Geometry check sheet. Reference: the model listing, model coordinates, mm. Face numbers are marked on the shaded views. Round coordinates to 2 decimals unless told otherwise and drop trailing zeros. Loops run counter-clockwise (first coordinate to the right, second up) from the corner with the lowest first, then second, coordinate; pieces in that order, holes last. Notation, with made-up numbers: (-23, -4.5) -> (-17, -4.5) arc R24 ccw to (-17, 24.5) -> close; hole circle Ø3 at (-8, 45.25). An arc over 180 degrees is marked (long way). Use a Markdown table: item, result. Add a question column.
Q1. Sectioned sample at B-B, the plane z = 4.25. Enter the section's corners in (x, y), then the cut area to 3 significant figures.
Q2. Sectioned sample at C-C, the plane x = 0. Enter the section's corners in (y, z).
Q3. Release check for a two-part mould opening along X. For the marked faces 1, 2 and 3 record: released by +X, released by -X, zero draft, split by the parting line, or undercut.
Q4. Sectioned sample at D-D, the plane x = 2. Enter the section's corners in (y, z), then the cut area to 3 significant figures.
Q5. Material ranges on L1, parallel to Y at x = 0, z = 1.15; L2, parallel to X at y = -12, z = 2.8; L3, parallel to X at y = 9, z = 0.45, recorded low to high.
Q6. Sectioned sample at A-A, the plane y = -10. Enter the section's corners in (x, z).
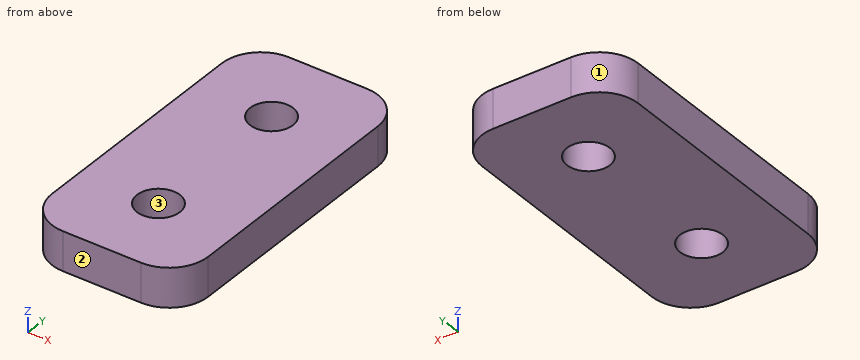
```python
from build123d import *

# Parameters (mm, degrees)
F0_W     = 20
F0_H     = 40
F0_R     = 2.75
F1_DEPTH = 5
F2_R     = 5


with BuildPart() as f1:
    # F0 (on Top) → F1 (new body)
    with BuildSketch(Plane.XY):
        Rectangle(F0_W, F0_H)
        with Locations((0, -10)):
            Circle(F0_R, mode=Mode.SUBTRACT)
        with Locations((0, 10)):
            Circle(F0_R, mode=Mode.SUBTRACT)
    extrude(amount=F1_DEPTH)

    # F2
    f2_edges = [f1.edges().sort_by_distance(p)[0] for p in [
        (-10, 20, 2.5),
        (10, 20, 2.5),
        (10, -20, 2.5),
        (-10, -20, 2.5),
    ]]
    fillet(f2_edges, radius=F2_R)


solid = f1.part
```
Values:
| question | item | result |
|---|---|---|
| 1 | outline | (-10, -15) arc R5 ccw to (-5, -20) -> (5, -20) arc R5 ccw to (10, -15) -> (10, 15) arc R5 ccw to (5, 20) -> (-5, 20) arc R5 ccw to (-10, 15) -> close; hole circle Ø5.5 at (0, -10); hole circle Ø5.5 at (0, 10) |
| 1 | area | 731 mm^2 |
| 2 | outline | (-20, 0) -> (-12.75, 0) -> (-12.75, 5) -> (-20, 5) -> close; (-7.25, 0) -> (7.25, 0) -> (7.25, 5) -> (-7.25, 5) -> close; (12.75, 0) -> (20, 0) -> (20, 5) -> (12.75, 5) -> close |
| 3 | face 1 | released by -X |
| 3 | face 2 | zero draft |
| 3 | face 3 | undercut |
| 4 | outline | (-20, 0) -> (-11.89, 0) -> (-11.89, 5) -> (-20, 5) -> close; (-8.11, 0) -> (8.11, 0) -> (8.11, 5) -> (-8.11, 5) -> close; (11.89, 0) -> (20, 0) -> (20, 5) -> (11.89, 5) -> close |
| 4 | area | 162 mm^2 |
| 5 | L1 | -20 to -12.75, -7.25 to 7.25, 12.75 to 20 |
| 5 | L2 | -10 to -1.89, 1.89 to 10 |
| 5 | L3 | -10 to -2.56, 2.56 to 10 |
| 6 | outline | (-10, 0) -> (-2.75, 0) -> (-2.75, 5) -> (-10, 5) -> close; (2.75, 0) -> (10, 0) -> (10, 5) -> (2.75, 5) -> close |
